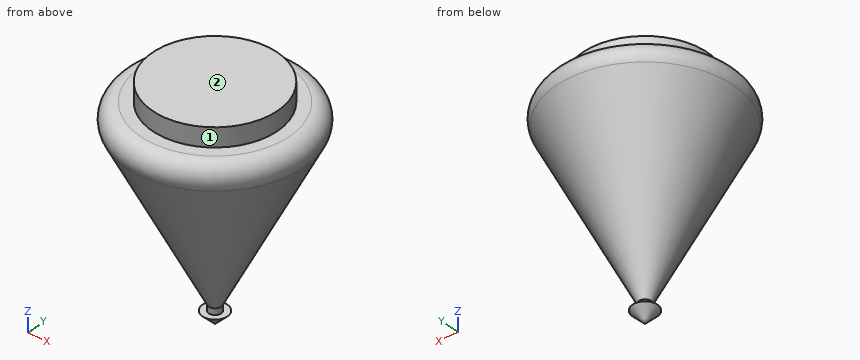
```python
from build123d import *


with BuildPart() as f1:
    # F0 (on Front) → F1 (revolve)
    with BuildSketch(Plane.XZ):
        with BuildLine():
            Line((50, -15), (50, 0))
            Line((50, 0), (0, 0))
            Line((0, 0), (0, -179.9984))
            Line((0, -179.9984), (10, -169.9984))
            Line((10, -169.9984), (5, -169.9984))
            Line((5, -169.9984), (5, -164.9984))
            Line((5, -164.9984), (70.810071, -33.379661))
            ThreePointArc((70.810071, -33.379661), (70.25415, -21.023238), (59.45087, -15))
            Line((59.45087, -15), (50, -15))
        make_face()
    revolve(axis=Axis((0, 0, -89.9992), (0, 0, -1)))


solid = f1.part
```
Model file for the job. Use its own axes, mm. Face numbers are marked on the shaded views. A direction names the side the tool comes from. Coordinates: 2 decimals unless noted, no trailing zeros. Loops run counter-clockwise (first coordinate to the right, second up) from the corner with the lowest first, then second, coordinate; pieces in that order, holes last. Notation, with made-up numbers: (72.25, 73.25) - (92.25, 73.25) arc R18 ccw to (92.25, 79.25) - close; hole circle Ø6 at (57.25, 29). An arc over 180 degrees is marked (long way). Write item = value, one per line. Start each with the question number.
Item 1: Saw through at B-B, the plane z = -107. List the corners of the cut face in (x, y), then the cut area to 3 significant figures.
Item 2: Wall check: probe 1 along X at (y, z) = (-2, -9.5); probe 2 along Z at (x, y) = (60, -3.5); probe 3 along Y at (x, z) = (-36, -34). Give the ranges that are in metal, low to high. Write a range as [from, to].
Item 3: Drop flat-ended pins along their axis: pin 1 Ø10 at (x, y) = (-25.5, -0.5) entering from -Z; pin 2 Ø3 at (y, z) = (-41, -73.5) entering from -X; pin 3 Ø2 at (x, z) = (-54, -30.5) entering from -Y. Give the stop position or say it passes through.
Item 4: 3-axis set-ups, long thin cutter, end or side, ignore diameter. For the marked faces 1 and 2: which of +Z, -Z, +X, -X, +Y, -Y reach the whole face in a straight line?
Item 5: Saw through at A-A, the plane z = -140.5. List the corners of the cut face in (x, y), then the cut area to 3 significant figures.
Answers:
q1.outline = circle Ø68 at (0, 0)
q1.area = 3,630 mm2
q2.probe_1 = [-49.96, 49.96]
q2.probe_2 = [-54.8, -15.02]
q2.probe_3 = [-60.62, 60.62]
q3.pin_1 = -133.99
q3.pin_2 = -32.21
q3.pin_3 = -48.54
q4.face_1 = +Z
q4.face_2 = +Z, +X, -X, +Y, -Y
q5.outline = circle Ø34.5 at (0, 0)
q5.area = 935 mm2
